Design review of the part built by this model. Coordinates are the model's own, in mm. Face numbers are marked on the shaded views. A direction names the side the tool comes from. Give positions to 0.01 mm unless a question says otherwise; leave off trailing zeros. Order: outer loops, then holes, each group sorted by start corner. A loop starts at its lowest first (then second) coordinate and runs counter-clockwise, first axis right, second up. Notation, with made-up numbers: (72.25, 60.25) -> (120.25, 60.25) arc R11 ccw to (120.25, 77.25) -> close; hole circle Ø9 at (45, 61.5). An arc over 180 degrees is marked (long way). One line per item, written item: value. Start each with the question number.
1) Consider section C-C (x = 26.25). State the section outline as (y, z) points, plus the area to 4 significant figures.
2) Consider section D-D (x = -41). State the section outline as (y, z) points.
3) Consider section A-A (x = 45.72). State the section outline as (y, z) points.
4) For pin 1 (3 mm diameter, centred on x = 26.25, z = -9.25, fed in from +Y) (1 decimal); pin 2 (15 mm diameter, centred on x = 3, z = 8, fed in from +Y); pin 3 (5.5 mm diameter, centred on x = 39.37, y = 24.13, fed in from +Z); pin 4 (4.5 mm diameter, centred on x = 45.72, y = -24.13, fed in from -Z), all flat-tipped, find the tip position at first contact; note any pin that passes through.
5) Wall thickness on line 1 along X through (y, z) = (-33.9, -9.25); line 2 along X through (y, z) = (-24.13, 1.9); line 3 along Y through (x, z) = (45.72, 2.55): over which ranges is each line inside the solid? List them lowest first. Write a range as from..to.
6) Consider section B-B (z = -9.25). State the section outline as (x, y) points, plus the area to 3 significant figures.
7) Tool access review of the marked faces 1 and 2: name each direction out of +Z, -Z, +X, -X, +Y, -Y from which nothing blocks a thin tool from reaching the whole face with its end or side.
Autodesk Inventor part; units mm, degrees
ref_plane "YZ Plane" through (0, 0, 0) normal (1, 0, 0) x (0, 1, 0)
ref_plane "XZ Plane" through (0, 0, 0) normal (0, 1, 0) x (-1, 0, 0)
ref_plane "XY Plane" through (0, 0, 0) normal (0, 0, 1) x (1, 0, 0)
sketch "Sketch1" plane through (0, 0, 0) normal (0, 0, 1) x (1, 0, 0)
  line L0 (-52.5, 32.5) -> (52.5, 32.5)
  line L1 (52.5, 32.5) -> (52.5, -32.5)
  line L2 (52.5, -32.5) -> (-52.5, -32.5)
  line L3 (-52.5, -32.5) -> (-52.5, 32.5)
  line L4 (-52.5, 32.5) -> (52.5, -32.5) construction
  line L5 (52.5, 32.5) -> (-52.5, -32.5) construction
  point P0 (0, 0)
  dimension "d0" = 105
  dimension "d1" = 65
extrude "Extrusion1" add sketch "Sketch1" along normal blind 3
sketch "Sketch2" plane through (0, 0, 3) normal (0, 0, 1) x (1, 0, 0)
  line L0 (-50.8, 26.67) -> (50.8, 26.67)
  line L1 (50.8, 26.67) -> (50.8, -26.67)
  line L2 (50.8, -26.67) -> (-50.8, -26.67)
  line L3 (-50.8, -26.67) -> (-50.8, 26.67)
  line L4 (-50.8, 26.67) -> (50.8, -26.67) construction
  line L5 (50.8, 26.67) -> (-50.8, -26.67) construction
  line L6 (50.8, -24.13) -> (-50.8, -24.13)
  line L7 (-35.56, -26.67) -> (-35.56, 26.67)
  line L8 (50.8, 24.13) -> (-50.8, 24.13)
  circle A0 centre (-35.56, 24.13) radius 3
  line L9 (-36.83, -26.67) -> (-36.83, 26.67)
  circle A1 centre (-36.83, -24.13) radius 3
  line L10 (45.72, -26.67) -> (45.72, 26.67)
  circle A2 centre (45.72, -24.13) radius 3
  line L11 (15.24, -26.67) -> (15.24, 26.67)
  line L12 (50.8, -19.05) -> (-50.8, -19.05)
  circle A3 centre (15.24, -19.05) radius 3
  line L13 (39.37, -26.67) -> (39.37, 26.67)
  circle A4 centre (39.37, 24.13) radius 3
  point P0 (0, 0)
  dimension "d4" = 101.6
  dimension "d5" = 53.34
  dimension "d6" = 2.54
  dimension "d7" = 15.24
  dimension "d8" = 50.8
  dimension "d9" = 6
  dimension "d10" = 13.97
  dimension "d11" = 6
  dimension "d12" = 96.52
  dimension "d13" = 6
  dimension "d14" = 66.04
  dimension "d15" = 7.62
  dimension "d16" = 6
  dimension "d17" = 90.17
  dimension "d18" = 6
extrude "Extrusion2" add sketch "Sketch2" along normal blind 1.5 contours L0 A0 | L9 L8 A0 L0 | L0 L7 L8 L9 | L0 A0 L8 L7 | L9 A0 L8 | L8 L7 A0 L9 | L8 A0 L7 | A4 L0 | L0 L13 L8 A4 | A1 L7 L6 L9 | L9 L6 A1 | L0 A4 L8 L13 | L8 L13 A4 | A3 L12 L11 | L11 L12 A3 | A1 L6 L7 | L12 L11 A3 | L9 L2 A1 L6 | L6 L7 L2 L9 | L8 A4 L13 | L12 A3 L11 | L6 A1 L2 L7 | L2 A1 | A2 L6 L10 | L10 L6 A2 | L6 L10 L2 A2 | L6 A2 L2 L10 | L2 A2
sketch "Sketch3" plane through (-35.56, 24.13, 4.5) normal (0, 0, 1) x (1, 0, 0)
  circle A0 centre (74.93, 0) radius 3
  circle A1 centre (81.28, -48.26) radius 3
  circle A2 centre (50.8, -43.18) radius 3
  circle A3 centre (-1.27, -48.26) radius 3
  point P0 (35.56, -24.13)
  point P1 (0, 0)
hole "Hole1" at (-35.56, 24.13, 4.5) at (39.37, 24.13, 4.5) at (45.72, -24.13, 4.5) at (15.24, -19.05, 4.5) at (-36.83, -24.13, 4.5) direction (0, 0, -1) diameter 3.5 end through all
sketch "Sketch4" plane through (-52.5, -32.5, 0) normal (0, -1, 0) x (1, 0, 0)
  line L0 (0, 0) -> (0, 3)
  line L1 (0, 1.5) -> (105, 1.5)
  line L2 (105, 0) -> (105, 3)
  line L3 (0, 16.5) -> (105, 16.5)
  line L4 (105, 16.5) -> (105, -13.5)
  line L5 (105, -13.5) -> (0, -13.5)
  line L6 (0, -13.5) -> (0, 16.5)
  line L7 (0, 16.5) -> (105, -13.5) construction
  line L8 (105, 16.5) -> (0, -13.5) construction
  point P0 (52.5, 0)
  point P1 (52.5, 1.5)
  dimension "d29" = 30
extrude "Extrusion3" add sketch "Sketch4" along normal blind 3
chamfer "Chamfer1" distance 5 angle 45 1 edges at (0, -32.5, 0)
sketch "Sketch5" plane through (-52.5, -32.5, 0) normal (0, 1, 0) x (1, 0, 0)
  line L0 (105, 5) -> (105, 13.5)
  line L1 (105, 9.25) -> (0, 9.25)
  line L2 (0, -16.5) -> (0, 13.5)
  line L3 (0, 13.5) -> (105, 13.5)
  line L4 (52.5, 13.5) -> (52.5, 5)
  line L5 (105, 5) -> (0, 5)
  line L6 (78.75, 13.5) -> (78.75, 5)
  line L7 (26.25, 13.5) -> (26.25, 5)
  point P0 (52.5, 0)
  point P1 (78.75, 9.25)
  point P2 (26.25, 9.25)
  dimension "d36" = 26.25
  dimension "d37" = 26.25
hole "Hole2" at (26.25, -32.5, -9.25) at (-26.25, -32.5, -9.25) direction (0, -1, 0) diameter 5 end through all
fillet "Fillet2" radius 2 6 edges at (-52.5, 32.5, 1.5) (-52.5, -34, 16.5) (-52.5, -34, -13.5) (52.5, -34, -13.5) (52.5, -34, 16.5) (52.5, 32.5, 1.5)
properties part number "Eletronica - suporteArduino"
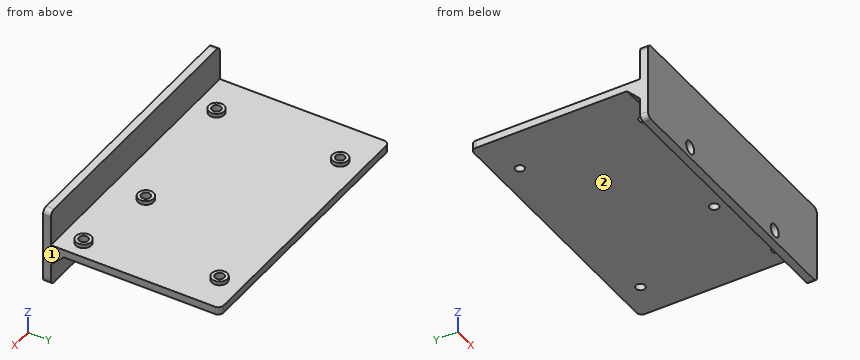
Checked values:
1. outline: (-35.5, -13.5) -> (-32.5, -13.5) -> (-32.5, -11.75) -> (-35.5, -11.75) -> close; (-35.5, -6.75) -> (-32.5, -6.75) -> (-32.5, -5) -> (-27.5, 0) -> (32.5, 0) -> (32.5, 3) -> (-32.5, 3) -> (-32.5, 16.5) -> (-35.5, 16.5) -> close
1. area: 282.5 mm^2
2. outline: (-35.5, -13.5) -> (-32.5, -13.5) -> (-32.5, -5) -> (-27.5, 0) -> (32.5, 0) -> (32.5, 3) -> (-32.5, 3) -> (-32.5, 16.5) -> (-35.5, 16.5) -> close
3. outline: (-35.5, -13.5) -> (-32.5, -13.5) -> (-32.5, -5) -> (-27.5, 0) -> (-25.88, 0) -> (-25.88, 4.5) -> (-27.13, 4.5) -> (-27.13, 3) -> (-32.5, 3) -> (-32.5, 16.5) -> (-35.5, 16.5) -> close; (-22.38, 0) -> (32.5, 0) -> (32.5, 3) -> (-21.13, 3) -> (-21.13, 4.5) -> (-22.38, 4.5) -> close
4. pin 1: passes through
4. pin 2: stops at y = 32.5
4. pin 3: stops at z = 4.5
4. pin 4: stops at z = 0
5. line 1: x = -52.5..-28.75, -23.75..23.75, 28.75..52.5
5. line 2: x = -52.5..-38.58, -35.08..43.97, 47.47..52.5
5. line 3: y = -35.5..-25.88, -22.38..32.5
6. outline: (-52.5, -35.5) -> (-28.75, -35.5) -> (-28.75, -32.5) -> (-52.5, -32.5) -> close; (-23.75, -35.5) -> (23.75, -35.5) -> (23.75, -32.5) -> (-23.75, -32.5) -> close; (28.75, -35.5) -> (52.5, -35.5) -> (52.5, -32.5) -> (28.75, -32.5) -> close
6. area: 285 mm^2
7. face 1: +Z, -Z, +X, +Y, -Y
7. face 2: -Z, +X, -X, +Y
